```python
from build123d import *

# Parameters (mm, degrees)
F0_W     = 128.39678
F0_H     = 128.39675
F1_DEPTH = 34.036
F2_R     = 43.0305
F3_DEPTH = 25.4
F4_R     = 36.680501
F5_DEPTH = 94.742


with BuildPart() as f1:
    # F0 (on Front) → F1 (new body)
    with BuildSketch(Plane.XZ):
        Rectangle(F0_W, F0_H)
    extrude(amount=F1_DEPTH)

    # F2 (on face) → F3 (join)
    with BuildSketch(Plane.XZ.offset(34.036)):
        Circle(F2_R)
    extrude(amount=F3_DEPTH)

    # F4 (on face) → F5 (cut)
    with BuildSketch(Plane.XZ.offset(59.436)):
        Circle(F4_R)
    extrude(amount=-F5_DEPTH, mode=Mode.SUBTRACT)


solid = f1.part
```
Geometry check sheet. Reference: the model listing, model coordinates, mm. A direction names the side the tool comes from. Give positions to 0.01 mm unless a question says otherwise; leave off trailing zeros. Write each loop counter-clockwise with the first axis right and the second up, starting at its lowest first coordinate (ties: lowest second). Pieces come first, ordered by that corner, then holes. Notation, with made-up numbers: (-16.5, 45) -> (4.5, 45) arc R35 cw to (4.5, 80) -> close; hole circle Ø3 at (10, 6.5). An arc over 180 degrees is marked (long way). Use one line per item in the form item = value.
Item 1: Mould release check, pull along Z, two halves, no side actions. Record for faces 1 (the cylindrical face through (-4.775, -30.134, 36.368)), 2 (the flat face through (-1, -17, -64.198)), 3 (the flat face through (-64.198, -17, -1)): released by +Z, released by -Z, zero draft, split by the parting line, or undercut.
Results list:
face_1 = undercut
face_2 = released by -Z
face_3 = zero draft
Item 2: Access from +Z, -Z, +X, -X, +Y, -Y to the whole of each face (thin tool, end or side, straight path). Record for faces 4 (the flat face through (-1, -34.036, 44)), 5 (the flat face through (-1, -17, 64.198)).
Results list:
face_4 = -Y
face_5 = +Z, +X, -X, +Y, -Y
Item 3: Sectioned sample at C-C on y = -5. Enter the section's corners in (x, z), plus the area to 3 significant figures.
Results list:
outline = (-64.2, -64.2) -> (64.2, -64.2) -> (64.2, 64.2) -> (-64.2, 64.2) -> close; hole circle Ø73.36 at (0, 0)
area = 12,300 mm2
Item 4: Sectioned sample at B-B on x = 0. Enter the section's corners in (y, z), plus the area to 3 significant figures.
Results list:
outline = (-59.44, -43.03) -> (-34.04, -43.03) -> (-34.04, -64.2) -> (0, -64.2) -> (0, -36.68) -> (-59.44, -36.68) -> close; (-59.44, 36.68) -> (0, 36.68) -> (0, 64.2) -> (-34.04, 64.2) -> (-34.04, 43.03) -> (-59.44, 43.03) -> close
area = 2,200 mm2
Item 5: Sectioned sample at A-A on z = 0. Enter the section's corners in (x, y), plus the area to 3 significant figures.
Results list:
outline = (-64.2, -34.04) -> (-43.03, -34.04) -> (-43.03, -59.44) -> (-36.68, -59.44) -> (-36.68, 0) -> (-64.2, 0) -> close; (36.68, -59.44) -> (43.03, -59.44) -> (43.03, -34.04) -> (64.2, -34.04) -> (64.2, 0) -> (36.68, 0) -> close
area = 2,200 mm2
Item 6: Sectioned sample at D-D on x = -53.5. Enter the section's corners in (y, z).
Results list:
outline = (-34.04, -64.2) -> (0, -64.2) -> (0, 64.2) -> (-34.04, 64.2) -> close
Item 7: Depth check by flat-ended pin: pin 1 Ø6 at (x, z) = (-36.5, 47) entering from -Y; pin 2 Ø1.5 at (y, z) = (-35.5, 48) entering from +X; pin 3 Ø10 at (x, y) = (0.5, -42) entering from +Z; pin 4 Ø1.5 at (x, y) = (-26.5, -39) entering from +Z. Enter the tip coordinate at first touch or a pass-through.
Results list:
pin_1 = -34.04
pin_2 = through
pin_3 = 43.03
pin_4 = 34.48
Item 8: Scan lines: line 1 (Z direction, x = 0, y = -22); line 2 (X direction, y = -4.5, z = 1.5); line 3 (Y direction, x = 29.5, z = 40). Record each from-to range of solid material in increasing order.
Results list:
line_1 = -64.2 to -36.68, 36.68 to 64.2
line_2 = -64.2 to -36.65, 36.65 to 64.2
line_3 = -34.04 to 0
